Geometry check sheet. Reference: the model listing, model coordinates, mm. A direction names the side the tool comes from. Give positions to 0.01 mm unless a question says otherwise; leave off trailing zeros. Write each loop counter-clockwise with the first axis right and the second up, starting at its lowest first coordinate (ties: lowest second). Pieces come first, ordered by that corner, then holes. Notation, with made-up numbers: (30.5, 5.5) - (78.5, 5.5) arc R16 cw to (78.5, 27.5) - close; hole circle Ø3 at (43.25, 6). An arc over 180 degrees is marked (long way). One line per question, with ' | ' between items. Start each with the question number.
Q1. Section check C-C on x = 26.5. Record the boundary of the cut face in (y, z), and give its area (3 significant figures).
Q2. Set-up check for faces 4 (the face through (-6.99, 13.85, 7.15)), 5 (the face through (-10, 14, -17)), 6 (the face through (2.05, 4.93, -15.616)), 7 (the face through (17, 14, 10)), 8 (the face through (11, 10, -11)): record each of +Z, -Z, +X, -X, +Y, -Y from which the full face is reachable in a straight line by a thin tool's end or side.
Q3. Section check A-A on y = 12.5. Record the boundary of the cut face in (x, z).
Q4. Section check D-D on z = -14. Record the boundary of the cut face in (x, y), and give its area (3 significant figures).
Q5. Thickness scan on L1, parallel to Y at x = 8, z = -18.5; L2, parallel to Z at x = 10.5, y = 11.25; L3, parallel to X at y = 4.5, z = -0.5. Record the ranges inside material, lowest first. Write a range as [from, to].
Q6. Gauge pin test, flat ends, axial feed: P1, Ø1, axis at y = 14.5, z = -11, coming from the +X side; P2, Ø1.5, axis at x = 15, y = 9.5, coming from the +Z side; P3, Ø1.5, axis at y = 7.5, z = -28.5, coming from the -X side; P4, Ø1.1, axis at x = 11, z = -11, coming from the +Y side. Record the tip position at first contact, or that the pin passes through.
Q7. Section check B-B on z = -4.5. Record the boundary of the cut face in (x, y).
Q8. Release check for a two-part mould opening along Y. For faces 1 (the face through (22, 14, -10)), 2 (the face through (-6, 10, 9)), 3 (the face through (0, 10, -24)) record: +Y half, -Y half, draft (parallel to the pull), parting line (faces both ways), or undercut.
Autodesk Inventor part; units mm, degrees
ref_plane "YZ Plane" through (0, 0, 0) normal (1, 0, 0) x (0, 1, 0)
ref_plane "XZ Plane" through (0, 0, 0) normal (0, 1, 0) x (-1, 0, 0)
ref_plane "XY Plane" through (0, 0, 0) normal (0, 0, 1) x (1, 0, 0)
sketch "Sketch1" plane through (0, 0, 0) normal (0, 1, 0) x (-1, 0, 0)
  circle A0 centre (0, 0) radius 15.75
  dimension "d0" = 31.5
extrude "Extrusion1" add sketch "Sketch1" along normal blind 10
sketch "Sketch2" plane through (0, 10, 0) normal (0, 1, 0) x (1, 0, 0)
  circle A0 centre (0, 0) radius 10
  line L0 (0, -10) -> (34, -10)
  line L1 (-10, 0) -> (-10, 34)
  line L2 (0, 10) -> (34, 10)
  line L3 (10, 0) -> (10, 34)
  line L4 (-8, 36) -> (8, 36)
  line L5 (36, -8) -> (36, 8)
  arc A1 (34, -10) -> (36, -8) centre (34, -8) ccw
  arc A2 (36, 8) -> (34, 10) centre (34, 8) ccw
  arc A3 (10, 34) -> (8, 36) centre (8, 34) ccw
  arc A4 (-8, 36) -> (-10, 34) centre (-8, 34) ccw
  point P0 (36, -10)
  point P1 (-10, 36)
  point P2 (10, 10)
  dimension "d3" = 20
  dimension "d4" = 36
  dimension "d5" = 36
  dimension "d6" = 2
  dimension "d7" = 20
  dimension "d8" = 20
extrude "Extrusion2" add sketch "Sketch2" along normal blind 7.8
properties part number "Door Lock"
Working result:
1) outline: (10, -10) - (17.8, -10) - (17.8, 10) - (10, 10) - close | area: 156 mm2
2) face 4: +Z, -X, +Y | face 5: +Z, -Z, -X, +Y | face 6: -Y | face 7: +Z, +X, -X, +Y | face 8: -Z, +X, +Y
3) outline: (-10, -34) arc R2 ccw to (-8, -36) - (8, -36) arc R2 ccw to (10, -34) - (10, -10) - (34, -10) arc R2 ccw to (36, -8) - (36, 8) arc R2 ccw to (34, 10) - (0, 10) arc R10 ccw to (-10, 0) - close
4) outline: (-10, 10) - (-7.22, 10) - (-7.22, 0) - (7.22, 0) - (7.22, 10) - (10, 10) - (10, 17.8) - (-10, 17.8) - close | area: 300 mm2
5) L1: y = [10, 17.8] | L2: z = [-10, 10] | L3: x = [-15.74, 15.74]
6) P1: stops at x = 10 | P2: stops at z = 10 | P3: passes through | P4: stops at y = 10
7) outline: (-15.09, 0) - (15.09, 0) - (15.09, 10) - (36, 10) - (36, 17.8) - (-10, 17.8) - (-10, 10) - (-15.09, 10) - close
8) face 1: draft | face 2: +Y half | face 3: -Y half
